Autodesk Inventor part; units mm, degrees
ref_plane "YZ Plane" through (0, 0, 0) normal (1, 0, 0) x (0, 1, 0)
ref_plane "XZ Plane" through (0, 0, 0) normal (0, 1, 0) x (-1, 0, 0)
ref_plane "XY Plane" through (0, 0, 0) normal (0, 0, 1) x (1, 0, 0)
sketch "Sketch1" plane through (0, 0, 0) normal (0, 1, 0) x (-1, 0, 0)
  circle A0 centre (0, 0) radius 5
  dimension "d0" = 10
extrude "Extrusion1" add sketch "Sketch1" along normal blind 4
sketch "Sketch2" plane through (0, 4, 0) normal (0, 1, 0) x (1, 0, 0)
  circle A0 centre (0, 0) radius 3
  dimension "d3" = 6
extrude "Extrusion2" add sketch "Sketch2" along normal blind 60
thread "Thread1"
sketch "Sketch3" plane through (0, 0, 0) normal (0, -1, 0) x (1, 0, 0)
  line L0 (-0.75, -10) -> (0.75, -10)
  line L1 (0.75, -10) -> (0.75, 10)
  line L2 (0.75, 10) -> (-0.75, 10)
  line L3 (-0.75, 10) -> (-0.75, -10)
  circle A0 centre (0, 0) radius 3
  line L4 (-0.75, -10) -> (0.75, 10) construction
  line L5 (0.75, -10) -> (-0.75, 10) construction
  dimension "d8" = 1.5
  dimension "d9" = 20
extrude "Extrusion3" cut sketch "Sketch3" against normal blind 2 contours L3 A0 L1 L0 | L3 A0 L1 | L3 L2 L1 A0
properties part number "vijs"
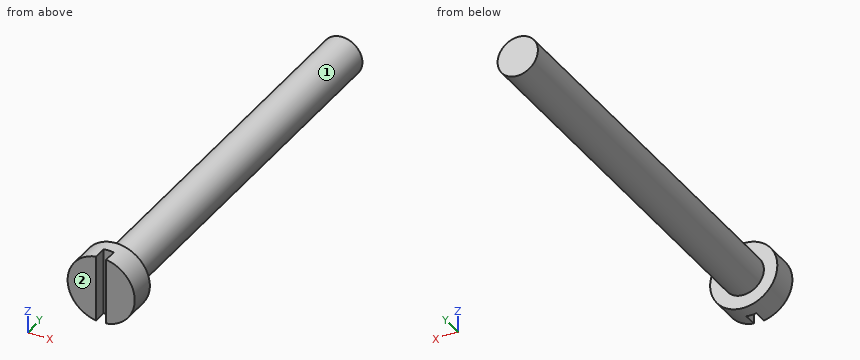
Can you work these out from the model? Positions are in its coordinate system, mm. Face numbers are marked on the shaded views. A direction names the side the tool comes from. Coordinates: 2 decimals unless noted, no trailing zeros. Write each loop counter-clockwise with the first axis right and the second up, starting at its lowest first coordinate (ties: lowest second). Pieces come first, ordered by that corner, then holes.
Q1. Imagine slicing it at A-A, the plane x = 0. List the corners of the cut face in (y, z) for me, plus the area to 3 significant figures.
Results found:
outline: (2, -5) - (4, -5) - (4, -3) - (64, -3) - (64, 3) - (4, 3) - (4, 5) - (2, 5) - close
area: 380 mm2
Q2. For P1, Ø4, axis at x = -3.5, y = 50, coming from the -Z side; P2, Ø1.6, axis at y = 0.5, z = -1.5, coming from the +X side; P3, Ø3, axis at x = 2.5, z = 1.5, coming from the -Y side; P4, Ø2, axis at x = 0, y = 25.5, coming from the -Z side, each with a flat end and sliding along its axis, tell me the tip position at first contact or that it passes through.
Results found:
P1: stops at z = -2.6
P2: stops at x = 4.95
P3: stops at y = 0
P4: stops at z = -3
Q3. Imagine slicing it at C-C, the plane y = 49.5. List the corners of the cut face in (x, z) for me, plus the area to 3 significant figures.
Results found:
outline: circle Ø6 at (0, 0)
area: 28.3 mm2
Q4. Imagine slicing it at B-B, the plane z = -4. List the corners of the cut face in (x, y) for me.
Results found:
outline: (-3, 0) - (-0.75, 0) - (-0.75, 2) - (0.75, 2) - (0.75, 0) - (3, 0) - (3, 4) - (-3, 4) - close
Q5. Please list where these lines run through material, in increasing order: L1, parallel to Y at x = -2.25, z = 3; L2, parallel to Z at x = 0.25, y = 6; L3, parallel to Y at x = -0.25, z = -2.25.
Results found:
L1: y = 0 to 4
L2: z = -2.99 to 2.99
L3: y = 2 to 64
Q6. Which directions (+Z, -Z, +X, -X, +Y, -Y) give clear straight access to the entire face, cutting with the end or side of a thin tool? Please do the marked faces 1 and 2.
Results found:
face 1: +Y
face 2: +Z, -Z, +X, -X, -Y
Q7. Imagine slicing it at D-D, the plane z = 0. List the corners of the cut face in (x, y) for me, plus the area to 3 significant figures.
Results found:
outline: (-5, 0) - (-0.75, 0) - (-0.75, 2) - (0.75, 2) - (0.75, 0) - (5, 0) - (5, 4) - (3, 4) - (3, 64) - (-3, 64) - (-3, 4) - (-5, 4) - close
area: 397 mm2
